Can you work these out from the drawing? Everything is in mm from the part's minimum corner. Round coordinates to 2 decimals unless told otherwise and drop trailing zeros. Write each loop counter-clockwise with the first axis right and the second up, starting at its lowest first coordinate (ties: lowest second). Pieces come first, ordered by that corner, then holes. Notation, with made-up numbers: (7, 15.5) -> (19, 15.5) arc R23 ccw to (19, 36.5) -> close; hole circle Ø3 at (20.25, 8). An arc over 180 degrees is marked (long way). Write item = value, one per line. Start each with the question number.
1) Imagine slicing it at D-D, the plane y = 13.5. Please give me the cut outline in (x, z).
2) Imagine slicing it at C-C, the plane x = 2.4. Please give me the cut outline in (y, z), then the cut area to 3 significant figures.
3) I'm going to push flat-ended pins straight in: pin 1 (1.8 mm diameter, centred on y = 31.5, z = 38.09, fed in from -X); pin 2 (1 mm diameter, centred on x = 2, z = 40, fed in from +Y); pin 3 (1 mm diameter, centred on x = 1.5, z = 39, fed in from -Y). Where does each tip first touch, or does it pass through?
4) If I drill on line 1 (Y direction, x = 1.9, z = 22.5); line 2 (Y direction, x = 0.4, z = 38) (1 decimal); line 3 (Z direction, x = 1.8, y = 13.5) (1 decimal), over which ranges is the centre line in solid material (lowest first)?
5) Imagine slicing it at A-A, the plane y = 40.5. Please give me the cut outline in (x, z).
6) Imagine slicing it at B-B, the plane z = 7. Please give me the cut outline in (x, y).
7) Thinking about a two-plate mould opening in Z: for the marked faces 1, 2 and 3, which applies, +Z half, -Z half, draft (parallel to the pull), parting line (faces both ways), or undercut?
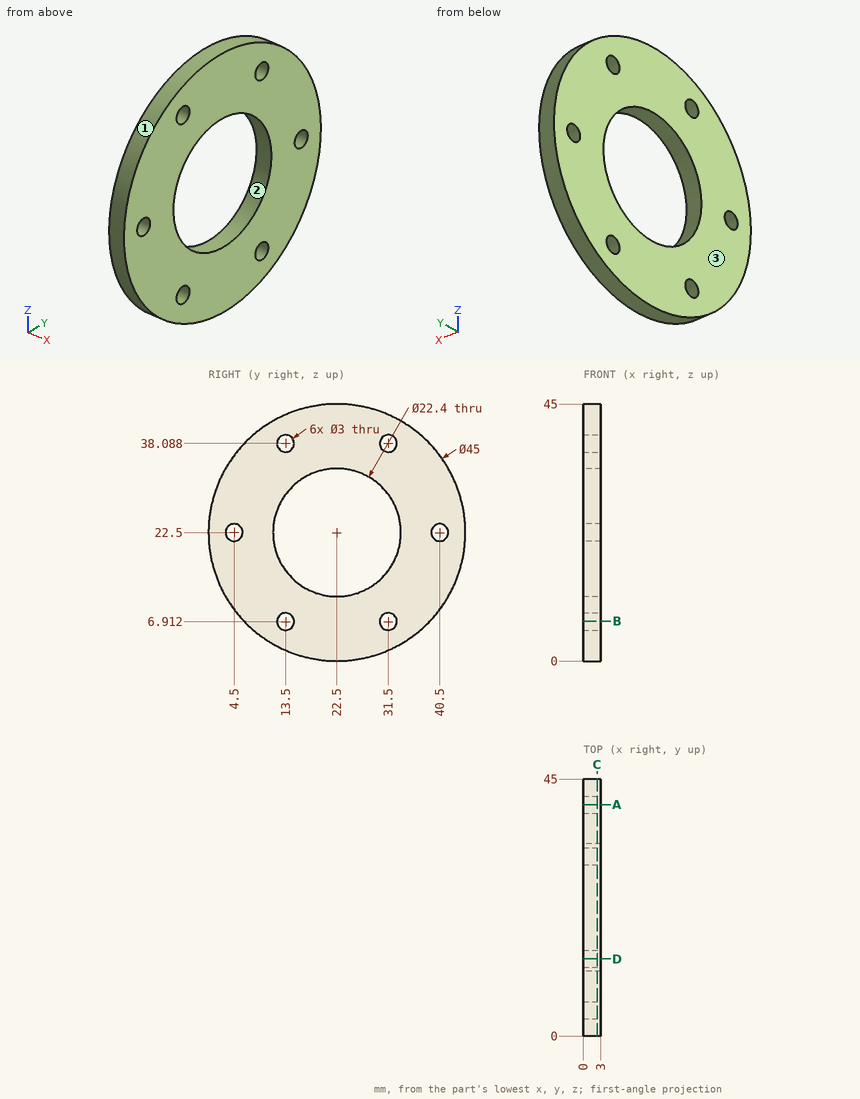
Reported:
q1.outline = (0, 1.88) -> (3, 1.88) -> (3, 5.41) -> (0, 5.41) -> close; (0, 8.41) -> (3, 8.41) -> (3, 15.83) -> (0, 15.83) -> close; (0, 29.17) -> (3, 29.17) -> (3, 36.59) -> (0, 36.59) -> close; (0, 39.59) -> (3, 39.59) -> (3, 43.12) -> (0, 43.12) -> close
q2.outline = circle Ø45 at (22.5, 22.5); hole circle Ø3 at (4.5, 22.5); hole circle Ø22.4 at (22.5, 22.5); hole circle Ø3 at (13.5, 6.91); hole circle Ø3 at (13.5, 38.09); hole circle Ø3 at (31.5, 6.91); hole circle Ø3 at (31.5, 38.09); hole circle Ø3 at (40.5, 22.5)
q2.area = 1,150 mm²
q3.pin_1 = through
q3.pin_2 = 37.24
q3.pin_3 = 6.68
q4.line_1 = 0 to 3, 6 to 11.3, 33.7 to 39, 42 to 45
q4.line_2 = 6.2 to 12, 15 to 30, 33 to 38.8
q4.line_3 = 1.9 to 5.4, 8.4 to 15.8, 29.2 to 36.6, 39.6 to 43.1
q5.outline = (0, 9) -> (3, 9) -> (3, 21) -> (0, 21) -> close; (0, 24) -> (3, 24) -> (3, 36) -> (0, 36) -> close
q6.outline = (0, 6.19) -> (3, 6.19) -> (3, 12) -> (0, 12) -> close; (0, 15) -> (3, 15) -> (3, 30) -> (0, 30) -> close; (0, 33) -> (3, 33) -> (3, 38.81) -> (0, 38.81) -> close
q7.face_1 = parting line
q7.face_2 = undercut
q7.face_3 = draft
